Part model, mm, in its own coordinate system. Face numbers are marked on the shaded views. A direction names the side the tool comes from. Coordinates: 2 decimals unless noted, no trailing zeros. Loops run counter-clockwise (first coordinate to the right, second up) from the corner with the lowest first, then second, coordinate; pieces in that order, holes last. Notation, with made-up numbers: (42.25, -25.75) - (77.25, -25.75) arc R18 cw to (77.25, -6.75) - close; hole circle Ø7 at (22.5, -32.75). An arc over 180 degrees is marked (long way). Use a Markdown table: item, result. Add a question column.
1. Pull direction Y, two halves, no side cores. Call the marked faces 1, 2, 3 and 4: pulls with the +Y half, pulls with the -Y half, needs draft (parallel to the pull), parting line crosses it, or undercut.
2. Wall check: probe 1 along Y at (x, z) = (0, 29.5) (3 decimals); probe 2 along Y at (x, z) = (-7.5, -11.5) (3 decimals); probe 3 along X at (y, z) = (56.5, 3) (3 decimals). Give the ranges that are in metal, low to high. Write a range as [from, to].
3. Band-saw the part on A-A, the plane z = 1.5. Give the cut face in (x, y) (3 decimals).
4. Band-saw the part on B-B, the plane y = 32. Give the cut face in (x, z) (3 decimals).
5. Band-saw the part on C-C, the plane x = -17.5. Give the cut face in (y, z) (3 decimals), plus the area to 3 significant figures.
6. Drop flat-ended pins along their axis: pin 1 (19 mm diameter, centred on y = 19, z = 8, fed in from -X); pin 2 (15 mm diameter, centred on x = 2, z = 7.5, fed in from +Y) (3 decimals); pin 3 (5 mm diameter, centred on x = -30, z = 28, fed in from -Y); pin 4 (3 mm diameter, centred on y = 57, z = -14.5, fed in from +X) (3 decimals). Give the stop position or say it passes through.
7. 3-axis set-ups, long thin cutter, end or side, ignore diameter. For the marked faces 5 and 6: which of +Z, -Z, +X, -X, +Y, -Y reach the whole face in a straight line?
8. Band-saw the part on D-D, the plane x = 41. Give the cut face in (y, z) (3 decimals).
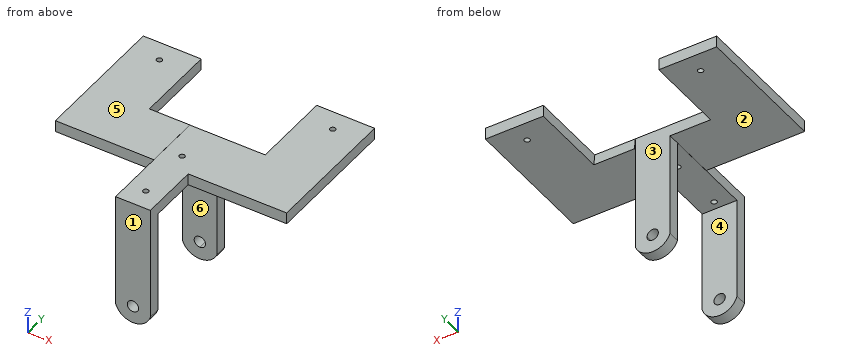
from build123d import *

# Parameters (mm, degrees)
F1_DEPTH  = 3.175
F2_DEPTH  = 3.175
F4_DEPTH  = 25.4
F5_DEPTH  = 25.4
F6_W      = 19.05
F6_H      = 63.5
F7_DEPTH  = 6.35
F9_DEPTH  = 6.35
F10_DEPTH = 2540
F11_R     = 1.5
F12_DEPTH = 25.4
F13_W     = 75.1403903484
F13_H     = 6.35
F14_DEPTH = 53.975
F15_R     = 1.5
F16_DEPTH = 25
F17_W     = 75.1403903484
F17_H     = 6.35
F18_DEPTH = 53.975
F19_R     = 1.5
F20_DEPTH = 25
F22_DEPTH = 22.225
F23_W     = 44.3243741632
F23_H     = 6.35
F24_DEPTH = 22.225


# Not quite as in the source:
# - a length typed as a fraction of an inch, garbled in the dataset ("3 / 203.2 mm" for 3/8 in), is restored


with BuildPart() as f1:
    # F0 (on Front) → F1 (new body)
    with BuildSketch(Plane.XZ):
        with BuildLine():
            Line((9.525, 25.206619263), (-9.525, 25.206619263))
            Line((-9.525, 25.206619263), (-9.525, -31.0143064708))
            ThreePointArc((-9.525, -31.0143064708), (0, -38.293380737), (9.525, -31.0143064708))
            Line((9.525, -31.0143064708), (9.525, 25.206619263))
        make_face()
    extrude(amount=F1_DEPTH)

    # F0 (on Front) → F2 (join)
    with BuildSketch(Plane.XZ):
        with BuildLine():
            Line((9.525, 25.206619263), (-9.525, 25.206619263))
            Line((-9.525, 25.206619263), (-9.525, -31.0143064708))
            ThreePointArc((-9.525, -31.0143064708), (0, -38.293380737), (9.525, -31.0143064708))
            Line((9.525, -31.0143064708), (9.525, 25.206619263))
        make_face()
    extrude(amount=-F2_DEPTH)

    # F3 (on Front) → F4 (cut)
    with BuildSketch(Plane.XZ):
        with BuildLine():
            ThreePointArc((0, -31.845793884), (2.2001627497, -30.9344566337), (3.1115, -28.734293884))
            ThreePointArc((3.1115, -28.734293884), (-2.2001627497, -26.5341311344), (0, -31.845793884))
        make_face()
    extrude(amount=-F4_DEPTH, mode=Mode.SUBTRACT)

    # F3 (on Front) → F5 (cut)
    with BuildSketch(Plane.XZ):
        with BuildLine():
            ThreePointArc((0, -31.845793884), (2.2001627497, -30.9344566337), (3.1115, -28.734293884))
            ThreePointArc((3.1115, -28.734293884), (-2.2001627497, -26.5341311344), (0, -31.845793884))
        make_face()
    extrude(amount=F5_DEPTH, mode=Mode.SUBTRACT)

    # F6 (on face) → F7 (join)
    with BuildSketch(Plane.XY.offset(25.206619263)):
        with Locations((0, 28.575)):
            Rectangle(F6_W, F6_H)
    extrude(amount=F7_DEPTH)

    # F11 (on face) → F12 (cut)
    with BuildSketch(Plane.XY.offset(31.556619263)):
        with Locations((0, 7.825)):
            Circle(F11_R)
        with Locations((0, 38.7934744358)):
            Circle(F11_R)
    extrude(amount=-F12_DEPTH, mode=Mode.SUBTRACT)



with BuildPart() as f9:
    # F8 (on face) → F9 (new body)
    with BuildSketch(Plane(origin=(0, 60.325, 0), x_dir=(-1, 0, 0), z_dir=(0, 1, 0))):
        with BuildLine():
            Line((-9.525, 31.556619263), (-9.525, -31.943380737))
            ThreePointArc((-9.525, -31.943380737), (0, -38.6772559995), (9.525, -31.943380737))
            Line((9.525, -31.943380737), (9.525, 31.556619263))
            Line((9.525, 31.556619263), (-9.525, 31.556619263))
        make_face()
    extrude(amount=-F9_DEPTH)

    # F3 (on Front) → F10 (cut)
    with BuildSketch(Plane.XZ):
        with BuildLine():
            ThreePointArc((0, -31.845793884), (2.2001627497, -30.9344566337), (3.1115, -28.734293884))
            ThreePointArc((3.1115, -28.734293884), (-2.2001627497, -26.5341311344), (0, -31.845793884))
        make_face()
    extrude(amount=-F10_DEPTH, mode=Mode.SUBTRACT)


with BuildPart() as f1_1:
    add(f1.part)

    add(f9.part)  # F14 merges F9
    # F13 (on face) → F14 (join)
    with BuildSketch(Plane.YZ.offset(9.525)):
        with Locations((66.7548048258, 28.381619263)):
            Rectangle(F13_W, F13_H)
    extrude(amount=F14_DEPTH)

    # F15 (on face) → F16 (cut)
    with BuildSketch(Plane.XY.offset(31.556619263)):
        with Locations((47.625, 93.325)):
            Circle(F15_R)
    extrude(amount=-F16_DEPTH, mode=Mode.SUBTRACT)

    # F17 (on face) → F18 (join)
    with BuildSketch(Plane(origin=(-9.525, 0, 0), x_dir=(0, -1, 0), z_dir=(-1, 0, 0))):
        with Locations((-67.0791789889, 28.4469667822)):
            Rectangle(F17_W, F17_H)
    extrude(amount=F18_DEPTH)

    # F19 (on face) → F20 (cut)
    with BuildSketch(Plane.XY.offset(31.6219667822)):
        with Locations((-47.625, 93.6493741632)):
            Circle(F19_R)
    extrude(amount=-F20_DEPTH, mode=Mode.SUBTRACT)

    # F21 (on face) → F22 (cut)
    with BuildSketch(Plane(origin=(9.525, 0, 0), x_dir=(0, -1, 0), z_dir=(-1, 0, 0))):
        Polygon((-104.325, 31.556619263), (-104.325, 25.206619263), (-61.1199513078, 25.206619263), (-60.325, 31.556619263), align=None)
    extrude(amount=-F22_DEPTH, mode=Mode.SUBTRACT)

    # F23 (on face) → F24 (cut)
    with BuildSketch(Plane.YZ.offset(-9.525)):
        with Locations((82.4871870816, 28.4469667822)):
            Rectangle(F23_W, F23_H)
    extrude(amount=-F24_DEPTH, mode=Mode.SUBTRACT)


solid = f1_1.part
Geometry check:
| question | item | result |
|---|---|---|
| 1 | face 1 | pulls with the -Y half |
| 1 | face 2 | needs draft |
| 1 | face 3 | pulls with the +Y half |
| 1 | face 4 | undercut |
| 2 | probe 1 | y = [-3.175, 6.325], [9.325, 37.293], [40.293, 60.325] |
| 2 | probe 2 | y = [-3.175, 3.175], [53.975, 60.325] |
| 2 | probe 3 | x = [-9.525, 9.525] |
| 3 | outline | (-9.525, -3.175) - (9.525, -3.175) - (9.525, 3.175) - (-9.525, 3.175) - close; (-9.525, 53.975) - (9.525, 53.975) - (9.525, 60.325) - (-9.525, 60.325) - close |
| 4 | outline | (-63.5, 25.272) - (-9.525, 25.272) - (-9.525, 25.207) - (63.5, 25.207) - (63.5, 31.557) - (-9.525, 31.557) - (-9.525, 31.622) - (-63.5, 31.622) - close |
| 5 | outline | (29.509, 25.272) - (60.325, 25.272) - (60.325, 31.622) - (29.509, 31.622) - close |
| 5 | area | 196 mm^2 |
| 6 | pin 1 | passes through |
| 6 | pin 2 | stops at y = 60.325 |
| 6 | pin 3 | stops at y = 29.51 |
| 6 | pin 4 | stops at x = 9.525 |
| 7 | face 5 | +Z, +X, -X, +Y, -Y |
| 7 | face 6 | -Z, +X, -X |
| 8 | outline | (29.185, 25.207) - (104.325, 25.207) - (104.325, 31.557) - (29.185, 31.557) - close |
